from build123d import *

# Parameters (mm, degrees)
SKETCH1_R                       = 6.9453125
BOSS_EXTRUDE1_DEPTH             = 19.05
F_21_0_159_DIAMETER_HOLE1_D     = 4.0386
F_21_0_159_DIAMETER_HOLE1_DEPTH = 7.0000114
F_21_0_159_DIAMETER_HOLE1_TIP   = 1.213317848
SKETCH5_W                       = 1.35255
SKETCH5_H                       = 6.9453125


with BuildPart() as part:
    # Sketch1 → Boss-Extrude1 (new body)
    with BuildSketch(Plane(origin=(0, 0, 0), x_dir=(0, 0, -1), z_dir=(1, 0, 0))):
        with Locations(Location((0, 0, 0), (0, 0, 180))):
            Circle(SKETCH1_R)
    extrude(amount=BOSS_EXTRUDE1_DEPTH)

    # #21 (0.159) Diameter Hole1
    with Locations(Plane(origin=(19.05, 0, 0), x_dir=(0, 0, -1), z_dir=(1, 0, 0))):
        with Locations((0, 0)):
            Hole(F_21_0_159_DIAMETER_HOLE1_D / 2, depth=F_21_0_159_DIAMETER_HOLE1_DEPTH)
            with Locations((0, 0, -(F_21_0_159_DIAMETER_HOLE1_DEPTH + F_21_0_159_DIAMETER_HOLE1_TIP / 2))):  # 118° drill point
                Cone(0, F_21_0_159_DIAMETER_HOLE1_D / 2, F_21_0_159_DIAMETER_HOLE1_TIP, mode=Mode.SUBTRACT)

    # Sketch5 → #6-32 Tapped Hole1 (revolve, cut)
    with BuildSketch(Plane(origin=(15.05, 0, 0), x_dir=(0, 0, -1), z_dir=(1, 0, 0))):
        with Locations((0.676275, 3.47265625)):
            Rectangle(SKETCH5_W, SKETCH5_H)
    revolve(axis=Axis((15.05, -6.35, 0), (0, 1, 0)), mode=Mode.SUBTRACT)


solid = part.part
Read the model definition and answer for the solid it produces. Units are mm, in the model's axes. A direction names the side the tool comes from. Coordinates: 2 decimals unless noted, no trailing zeros. Loops run counter-clockwise (first coordinate to the right, second up) from the corner with the lowest first, then second, coordinate; pieces in that order, holes last. Notation, with made-up numbers: (-26.5, -13.75) -> (28.5, -13.75) arc R8 ccw to (28.5, -5.75) -> close; hole circle Ø6 at (33.5, 11). An arc over 180 degrees is marked (long way). Write item = value, one per line. Start each with the question number.
1) The part is cut by section A-A, the plane x = 17.25. Determine the outline of the cut face in (y, z), plus the area to 3 significant figures.
2) For faces 4 (the face through (0, 0, 0)), 5 (the face through (14.99, 4.26, 1.35)), determine the directions among +Z, -Z, +X, -X, +Y, -Y from which every point of the face is accessible in a straight line to the end or side of a thin tool.
3) Given P1, Ø2.5, axis at y = 0, z = 0, coming from the +X side; P2, Ø8, axis at x = 13.5, z = -5.5, coming from the +Y side; P3, Ø3, axis at x = 15, y = 2.5, coming from the -Z side, each flat-ended and moving along its own axis, determine where each tip first touches the part or whether it passes through.
4) The part is cut by section C-C, the plane x = 6. Determine the outline of the cut face in (y, z), plus the area to 3 significant figures.
5) Find the intervals of material crossed by L1, parallel to X at y = 3.6, z = 0; L2, parallel to Y at x = 17, z = 0; L3, parallel to Z at x = 2, y = -0.25, in increasing order. Write a range as from..to.
6) The mould has two halves that part along Z. Classify faces 1 (the face through (19.05, 1, -2)), 2 (the face through (15.5, -1.97, -0.44)), 3 (the face through (9.392, -6.886, -0.904)): pulls with the +Z half, pulls with the -Z half, needs draft (parallel to the pull), parting line crosses it, or undercut.
7) The part is cut by section D-D, the plane z = -2.75. Determine the outline of the cut face in (x, y), plus the area to 3 significant figures.
8) The part is cut by section B-B, the plane y = 4.5. Determine the outline of the cut face in (x, z), plus the area to 3 significant figures.
Result:
q1.outline = circle Ø13.89 at (0, 0); hole circle Ø4.04 at (0, 0)
q1.area = 139 mm²
q2.face_4 = +Z, -Z, -X, +Y, -Y
q2.face_5 = +Y
q3.P1 = 11.59
q3.P2 = 6.78
q3.P3 = -6.87
q4.outline = circle Ø13.89 at (0, 0)
q4.area = 152 mm²
q5.L1 = 0..13.7, 16.4..19.05
q5.L2 = -6.95..-2.02, 2.02..6.95
q5.L3 = -6.94..6.94
q6.face_1 = needs draft
q6.face_2 = undercut
q6.face_3 = parting line crosses it
q7.outline = (0, -6.38) -> (19.05, -6.38) -> (19.05, 6.38) -> (0, 6.38) -> close
q7.area = 243 mm²
q8.outline = (0, -5.29) -> (19.05, -5.29) -> (19.05, 5.29) -> (0, 5.29) -> close; hole circle Ø2.71 at (15.05, 0)
q8.area = 196 mm²
